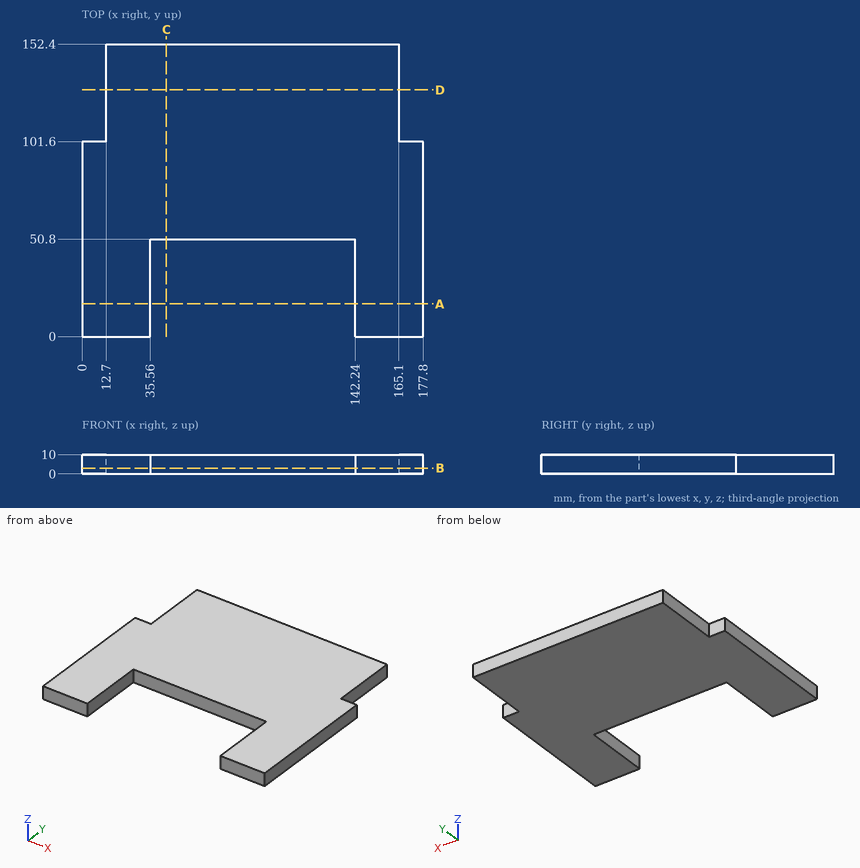
Geometry check sheet. Reference: drawing and pictorial views, mm from the part's lowest x, y, z. Coordinates: 2 decimals unless noted, no trailing zeros. Order: outer loops, then holes, each group sorted by start corner. A loop starts at its lowest first (then second) coordinate and runs counter-clockwise, first axis right, second up.
Item 1: Section check A-A (y = 17). Enter the section's corners in (x, z), plus the area to 3 significant figures.
Item 2: Section check B-B (z = 3). Enter the section's corners in (x, y), plus the area to 3 significant figures.
Item 3: Section check C-C (x = 44). Enter the section's corners in (y, z).
Item 4: Section check D-D (y = 128.5). Enter the section's corners in (x, z).
Item 5: Depth check by flat-ended pin: pin 1 (5 mm diameter, centred on y = 132, z = 4, fed in from -X); pin 2 (6 mm diameter, centred on y = 125.5, z = 4, fed in from +X); pin 3 (1.5 mm diameter, centred on x = 85.5, z = 8, fed in from -Y). Enter the tip coordinate at first touch or a pass-through.
Item 6: Scan lines: line 1 along X through (y, z) = (16.5, 3); line 2 along Y through (x, z) = (58.5, 5.5); line 3 along Y through (x, z) = (7, 8). Record each from-to range of solid material in increasing order.
Check sheet entries:
1. outline: (0, 0) - (35.56, 0) - (35.56, 10) - (0, 10) - close; (142.24, 0) - (177.8, 0) - (177.8, 10) - (142.24, 10) - close
1. area: 711 mm2
2. outline: (0, 0) - (35.56, 0) - (35.56, 50.8) - (142.24, 50.8) - (142.24, 0) - (177.8, 0) - (177.8, 101.6) - (165.1, 101.6) - (165.1, 152.4) - (12.7, 152.4) - (12.7, 101.6) - (0, 101.6) - close
2. area: 20,400 mm2
3. outline: (50.8, 0) - (152.4, 0) - (152.4, 10) - (50.8, 10) - close
4. outline: (12.7, 0) - (165.1, 0) - (165.1, 10) - (12.7, 10) - close
5. pin 1: stops at x = 12.7
5. pin 2: stops at x = 165.1
5. pin 3: stops at y = 50.8
6. line 1: x = 0 to 35.56, 142.24 to 177.8
6. line 2: y = 50.8 to 152.4
6. line 3: y = 0 to 101.6
